Input: part model. Units: mm. Frame: model coordinates. Face numbers are marked on the shaded views. A direction names the side the tool comes from. Round coordinates to 2 decimals unless told otherwise and drop trailing zeros. Loops run counter-clockwise (first coordinate to the right, second up) from the corner with the lowest first, then second, coordinate; pieces in that order, holes last.
(1) First-contact query: pin 1 Ø5 at (x, y) = (8, 11.5) entering from +Z; pin 2 Ø1.6 at (x, z) = (8, 7) entering from -Y. Flat tips, straight axial feed; report the tip coordinate or a pass-through.
(2) Cut plane A-A, the plane x = 20. Output: boundary loops of the cut face in (y, z), and give its area (3 significant figures).
(3) Draft query along Y for the marked faces 1, 2 and 3. Return one class per face: released by +Y, released by -Y, zero draft, split by the parting line, or undercut.
(4) Cut plane B-B, the plane y = 32. Output: boundary loops of the cut face in (x, z), and give its area (3 significant figures).
(5) Cut plane C-C, the plane x = 15. Output: boundary loops of the cut face in (y, z).
(6) Access query for the marked faces 4 and 5. Directions: +Z, -Z, +X, -X, +Y, -Y. A direction counts if a zero-diameter tool reaches every point of the face in a straight line with its end or side. Return the directions, or none.
(7) Line query: line 1 (Y direction, x = 18, z = 3.75); line 2 (X direction, y = 34.5, z = 8.25); line 3 (Y direction, x = 9.75, z = 2.75). Output: solid intervals per line, ascending.
from build123d import *

# Parameters (mm, degrees)
SKETCH_2_W           = 27
SKETCH_2_H           = 40
EXTRUDE_1_DEPTH      = 10
CUT_EXTRUDE_1_DEPTH  = 1.5
CUT_EXTRUDE_2_DEPTH  = 7.5
SKETCH_9_W           = 9
SKETCH_9_H           = 4.718038217
CUT_EXTRUDE_8_DEPTH  = 6.5
SKETCH_9_3_W         = 9
SKETCH_9_3_H         = 4.718038217
CUT_EXTRUDE_9_DEPTH  = 3.2
SKETCH_13_W          = 9
SKETCH_13_H          = 3.2
SKETCH_13_H_2        = 6.5
CUT_EXTRUDE_11_DEPTH = 3.281961783
CUT_EXTRUDE_12_REACH = 42
SKETCH_14_W          = 1.2
SKETCH_14_H          = 2.1
SKETCH_16_2_W        = 7
SKETCH_16_2_H        = 2.5
EXTRUDE_3_DEPTH      = 1
SKETCH_16_W          = 7
SKETCH_16_H          = 2.5
EXTRUDE_2_DEPTH      = 1
CUT_EXTRUDE_14_DEPTH = 2
SKETCH_18_W          = 12
SKETCH_18_H          = 3.3
CUT_EXTRUDE_15_DEPTH = 7
SKETCH_19_W          = 27
SKETCH_19_H          = 40
CUT_EXTRUDE_16_DEPTH = 0.5
FILLET_1_R           = 0.5
FILLET_2_R           = 0.5


with BuildPart() as part:
    # Sketch 2 → Extrude 1 (new body)
    with BuildSketch(Plane.XY):
        with Locations((13.5, 20)):
            Rectangle(SKETCH_2_W, SKETCH_2_H)
    extrude(amount=EXTRUDE_1_DEPTH)

    # Sketch 3 → Cut-Extrude 1 (cut)
    with BuildSketch(Plane.XY.offset(10)):
        with BuildLine():
            Line((1, 38), (1, 2))
            ThreePointArc((1, 2), (1.292893219, 1.292893219), (2, 1))
            Line((2, 1), (25, 1))
            ThreePointArc((25, 1), (25.707106781, 1.292893219), (26, 2))
            Line((26, 2), (26, 38))
            ThreePointArc((26, 38), (25.707106781, 38.707106781), (25, 39))
            Line((25, 39), (2, 39))
            ThreePointArc((2, 39), (1.292893219, 38.707106781), (1, 38))
        make_face()
    extrude(amount=-CUT_EXTRUDE_1_DEPTH, mode=Mode.SUBTRACT)

    # Sketch 5 → Cut-Extrude 2 (cut)
    with BuildSketch(Plane.XY.offset(8.5)):
        with BuildLine():
            Line((2, 39), (25, 39))
            ThreePointArc((25, 39), (25.707106781, 38.707106781), (26, 38))
            Line((26, 38), (26, 8))
            Line((26, 8), (1, 8))
            Line((1, 8), (1, 38))
            ThreePointArc((1, 38), (1.292893219, 38.707106781), (2, 39))
        make_face()
    extrude(amount=-CUT_EXTRUDE_2_DEPTH, mode=Mode.SUBTRACT)

    # Sketch 9 → Cut-Extrude 8 (cut)
    with BuildSketch(Plane.XY.offset(8.5)):
        with Locations((20.5, 4.640980891)):
            Rectangle(SKETCH_9_W, SKETCH_9_H)
    extrude(amount=-CUT_EXTRUDE_8_DEPTH, mode=Mode.SUBTRACT)

    # Sketch 9_3 → Cut-Extrude 9 (cut)
    with BuildSketch(Plane.XY.offset(8.5)):
        with Locations((6.5, 4.640980891)):
            Rectangle(SKETCH_9_3_W, SKETCH_9_3_H)
    extrude(amount=-CUT_EXTRUDE_9_DEPTH, mode=Mode.SUBTRACT)

    # Sketch 13 → Cut-Extrude 11 (cut, through all)
    with BuildSketch(Plane(origin=(0, 2.281961783, 0), x_dir=(1, 0, 0), z_dir=(0, 1, 0))):
        with Locations((6.5, -6.9)):
            Rectangle(SKETCH_13_W, SKETCH_13_H)
        with Locations((20.5, -5.25)):
            Rectangle(SKETCH_13_W, SKETCH_13_H_2)
    extrude(amount=-CUT_EXTRUDE_11_DEPTH, mode=Mode.SUBTRACT)

    # Sketch 14 → Cut-Extrude 12 (cut, up to next)
    with BuildSketch(Plane.XZ, mode=Mode.PRIVATE) as cut_extrude_12_sk1:
        with BuildLine():
            Line((12.9, 7.9), (14.1, 7.9))
            ThreePointArc((14.1, 7.9), (13.5, 7.3), (12.9, 7.9))
        make_face()
    cut_extrude_12_tool1 = extrude(cut_extrude_12_sk1.sketch, amount=-CUT_EXTRUDE_12_REACH, mode=Mode.PRIVATE) & part.part
    add(cut_extrude_12_tool1.solids().sort_by_distance((13.5, 0, 7.645352))[0], mode=Mode.SUBTRACT)
    # Sketch 14 → Cut-Extrude 12 (cut, up to next)
    with BuildSketch(Plane.XZ, mode=Mode.PRIVATE) as cut_extrude_12_sk2:
        with Locations((13.5, 8.95)):
            Rectangle(SKETCH_14_W, SKETCH_14_H)
    cut_extrude_12_tool2 = extrude(cut_extrude_12_sk2.sketch, amount=-CUT_EXTRUDE_12_REACH, mode=Mode.PRIVATE) & part.part
    add(cut_extrude_12_tool2.solids().sort_by_distance((13.5, 0, 8.95))[0], mode=Mode.SUBTRACT)

    # Sketch 16_2 → Extrude 3 (add)
    with BuildSketch(Plane.XZ.offset(-39)):
        with Locations((13.5, 7.25)):
            Rectangle(SKETCH_16_2_W, SKETCH_16_2_H)
    extrude(amount=EXTRUDE_3_DEPTH)

    # Sketch 16 → Extrude 2 (add)
    with BuildSketch(Plane.XZ.offset(-39)):
        with Locations((13.5, 7.25)):
            Rectangle(SKETCH_16_W, SKETCH_16_H)
    extrude(amount=EXTRUDE_2_DEPTH)

    # Sketch 17 → Cut-Extrude 14 (cut)
    with BuildSketch(Plane(origin=(0, 40, 0), x_dir=(1, 0, 0), z_dir=(0, 1, 0))):
        with BuildLine():
            Line((14.25, -7.75), (14.25, -10))
            Line((14.25, -10), (12.75, -10))
            Line((12.75, -10), (12.75, -7.75))
            ThreePointArc((12.75, -7.75), (13.5, -7), (14.25, -7.75))
        make_face()
    extrude(amount=-CUT_EXTRUDE_14_DEPTH, mode=Mode.SUBTRACT)

    # Sketch 18 → Cut-Extrude 15 (cut)
    with BuildSketch(Plane(origin=(0, 8, 0), x_dir=(1, 0, 0), z_dir=(0, 1, 0))):
        with Locations((7, -2.65)):
            Rectangle(SKETCH_18_W, SKETCH_18_H)
    extrude(amount=-CUT_EXTRUDE_15_DEPTH, mode=Mode.SUBTRACT)

    # Sketch 19 → Cut-Extrude 16 (cut)
    with BuildSketch(Plane.XY.offset(10)):
        with Locations((13.5, 20)):
            Rectangle(SKETCH_19_W, SKETCH_19_H)
    extrude(amount=-CUT_EXTRUDE_16_DEPTH, mode=Mode.SUBTRACT)

    # Fillet 1
    fillet_1_edges = [part.edges().sort_by_distance(p)[0] for p in [
        (27, 40, 4.75),
        (0, 40, 4.75),
        (27, 0, 4.75),
        (0, 0, 4.75),
        (20.55, 0, 9.5),
        (20.625, 40, 9.5),
        (6.375, 40, 9.5),
        (0, 20, 9.5),
        (27, 20, 9.5),
        (6.45, 0, 9.5),
        (13.5, 40, 0),
        (27, 20, 0),
        (13.5, 0, 0),
        (0, 20, 0),
    ]]
    fillet(fillet_1_edges, radius=FILLET_1_R)

    # Fillet 2
    fillet_2_edges = [part.edges().sort_by_distance(p)[0] for p in [
        (11, 0, 6.9),
        (2, 0, 6.9),
        (6.5, 0, 5.3),
        (25, 0, 5.25),
        (16, 0, 5.25),
        (20.5, 0, 2),
    ]]
    fillet(fillet_2_edges, radius=FILLET_2_R)


solid = part.part
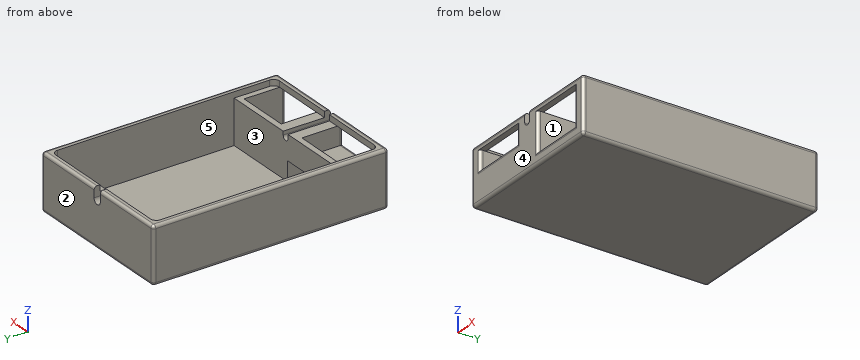
Reported:
1. pin 1: stops at z = 1
1. pin 2: stops at y = 7
2. outline: (0, 0.5) arc R0.5 ccw to (0.5, 0) - (39.5, 0) arc R0.5 ccw to (40, 0.5) - (40, 9) arc R0.5 ccw to (39.5, 9.5) - (39, 9.5) - (39, 1) - (8, 1) - (8, 8.5) - (7, 8.5) - (7, 2) - (0.5, 2) arc R0.5 ccw to (0, 1.5) - close; (0, 8.5) - (1, 8.5) - (1, 9.5) - (0.5, 9.5) arc R0.5 ccw to (0, 9) - close
2. area: 63.7 mm2
3. face 1: zero draft
3. face 2: released by +Y
3. face 3: undercut
4. outline: (0, 0.5) arc R0.5 ccw to (0.5, 0) - (26.5, 0) arc R0.5 ccw to (27, 0.5) - (27, 9) arc R0.5 ccw to (26.5, 9.5) - (26, 9.5) - (26, 1) - (1, 1) - (1, 9.5) - (0.5, 9.5) arc R0.5 ccw to (0, 9) - close
4. area: 43.8 mm2
5. outline: (0, 0.5) arc R0.5 ccw to (0.5, 0) - (39.5, 0) arc R0.5 ccw to (40, 0.5) - (40, 9) arc R0.5 ccw to (39.5, 9.5) - (39, 9.5) - (39, 8.5) - (38, 8.5) - (38, 6) - (39, 6) - (39, 1) - (8, 1) - (8, 8.5) - (1, 8.5) - (1, 9.5) - (0.5, 9.5) arc R0.5 ccw to (0, 9) - close
6. face 4: +Z, -Z, +X, -X, -Y
6. face 5: +Z
7. line 1: y = 7 to 8, 39 to 40
7. line 2: x = 0 to 1, 26 to 27
7. line 3: y = 0 to 1, 39 to 40
